Here's the drawing with two shaded views (mm, measured from the low corner). I have some questions. A direction names the side the tool comes from. Coordinates: 2 decimals unless noted, no trailing zeros. Loops run counter-clockwise (first coordinate to the right, second up) from the corner with the lowest first, then second, coordinate; pieces in that order, holes last. Notation, with made-up numbers: M 21.5,25 L 31.5,25 A36 cw 31.5,63 Z; hole C 48.5,75.5 d1. An arc over 180 degrees is marked long. Use one line per item in the form item = value. Start each with the question number.
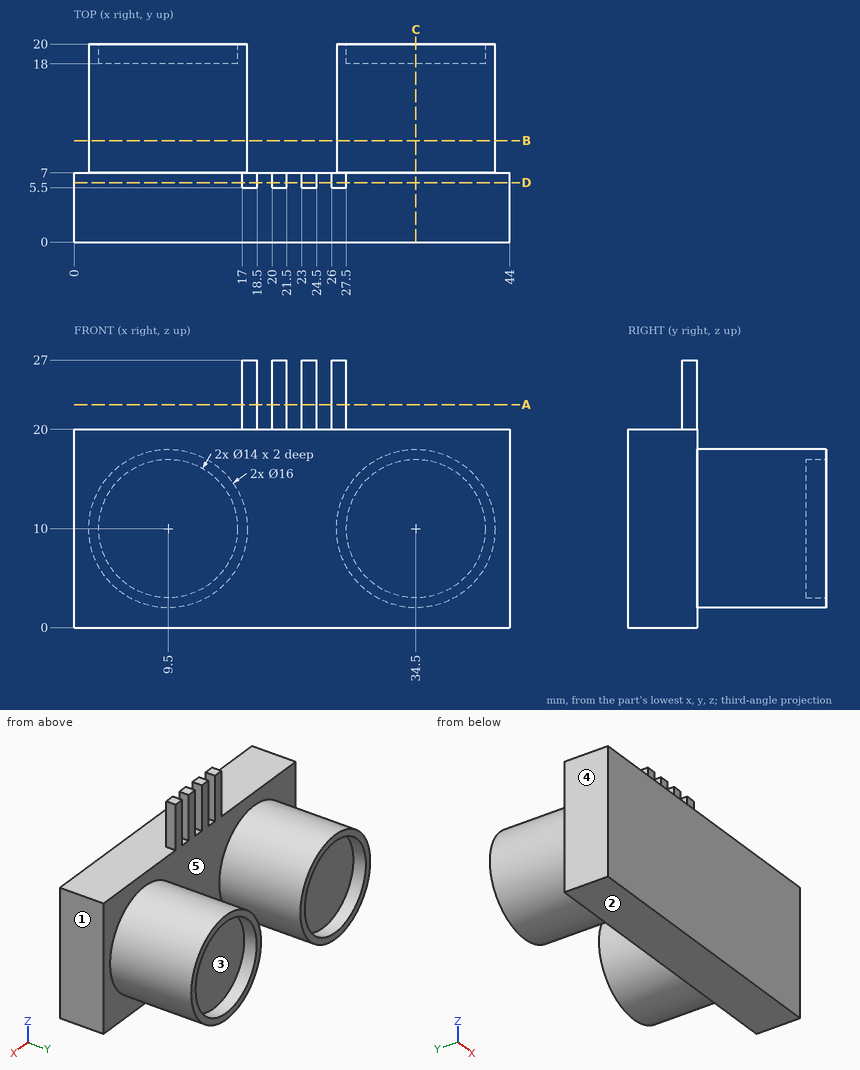
Item 1: I want a section at D-D (y = 6). Write out the boundary of the cut face in (x, z), plus the area to 3 significant figures.
Item 2: Please list where these lines run through material, in increasing order: line 1 along X through (y, z) = (19.2, 10); line 2 along Z through (x, y) = (9.5, 18.95); line 3 along Y through (x, z) = (24.5, 10.75).
Item 3: I want a section at B-B (y = 10.25). Write out the boundary of the cut face in (x, z).
Item 4: For the marked faces 4 and 5, which set-ups out of +Z, -Z, +X, -X, +Y, -Y let a thin tool reach every point of the face, with its end or its side?
Item 5: Thinking about a two-plate mould opening in X: for the marked faces 1, 2 and 3, which applies, pulls with the +X half, pulls with the -X half, needs draft (parallel to the pull), parting line crosses it, or undercut?
Item 6: I want a section at C-C (x = 34.5). Write out the boundary of the cut face in (y, z), plus the area to 3 significant figures.
Item 7: I'm going to push flat-ended pins straight in: P1, Ø12.5, axis at x = 9.5, z = 10, coming from the -Y side; P2, Ø3.5, axis at x = 13, y = 3.5, coming from the +Z side; P3, Ø1.5, axis at y = 11.5, z = 6.5, coming from the -X side; P4, Ø1, axis at y = 7, z = 22, coming from the +X side. Where does each tip first touch, or does it pass through?
Item 8: I want a section at A-A (z = 22.5). Write out the boundary of the cut face in (x, y).
Worked answers:
q1.outline = M 0,0 L 44,0 L 44,20 L 27.5,20 L 27.5,27 L 26,27 L 26,20 L 24.5,20 L 24.5,27 L 23,27 L 23,20 L 21.5,20 L 21.5,27 L 20,27 L 20,20 L 18.5,20 L 18.5,27 L 17,27 L 17,20 L 0,20 Z
q1.area = 922 mm²
q2.line_1 = 1.5 to 2.5, 16.5 to 17.5, 26.5 to 27.5, 41.5 to 42.5
q2.line_2 = 2 to 3, 17 to 18
q2.line_3 = 0 to 7
q3.outline = C 9.5,10 d16; C 34.5,10 d16
q4.face_4 = +Z, -Z, -X, +Y, -Y
q4.face_5 = +Y
q5.face_1 = pulls with the +X half
q5.face_2 = needs draft
q5.face_3 = undercut
q6.outline = M 0,0 L 7,0 L 7,2 L 20,2 L 20,3 L 18,3 L 18,17 L 20,17 L 20,18 L 7,18 L 7,20 L 0,20 Z
q6.area = 320 mm²
q7.P1 = 0
q7.P2 = 20
q7.P3 = 1.99
q7.P4 = 27.5
q8.outline = M 17,5.5 L 18.5,5.5 L 18.5,7 L 17,7 Z; M 20,5.5 L 21.5,5.5 L 21.5,7 L 20,7 Z; M 23,5.5 L 24.5,5.5 L 24.5,7 L 23,7 Z; M 26,5.5 L 27.5,5.5 L 27.5,7 L 26,7 Z
